Source: CAD feature listing. Evaluate the final solid. Frame: model axes, mm. Give positions to 0.01 mm unless a question says otherwise; leave off trailing zeros. Write each loop counter-clockwise with the first axis right and the second up, starting at its lowest first coordinate (ties: lowest second). Pieces come first, ordered by that corner, then holes. Notation, with made-up numbers: (73.5, 17.5) - (120.5, 17.5) arc R12 ccw to (120.5, 39.5) - close; hole circle Ø4 at (46.25, 23). An arc over 180 degrees is marked (long way). Answer as a JSON object with one key per item and string values. Group by question number.
from build123d import *

# Parameters (mm, degrees)
SKETCH_1_R          = 1.6
EXTRUDE_1_DEPTH     = 2
SKETCH_3_R          = 4.5
SKETCH_3_R_2        = 1.25
CUT_EXTRUDE_1_DEPTH = 3
CUT_EXTRUDE_2_DEPTH = 3
FILLET_1_R          = 1
SKETCH_5_R          = 33.5
CUT_EXTRUDE_3_DEPTH = 3


with BuildPart() as part:
    # ｽｹｯﾁ1 → ﾎﾞｽ - 押し出し1 (new body)
    with BuildSketch(Plane.XY):
        with BuildLine():
            Line((-3, -39.182266397), (-3, -41.291643997))
            Line((-3, -41.291643997), (3, -41.291643997))
            Line((3, -41.291643997), (3, -39.182266397))
            ThreePointArc((3, -39.182266397), (3.498945518, -37.860587373), (4.746835443, -37.198354174))
            ThreePointArc((4.746835443, -37.198354174), (26.516504294, -26.516504294), (37.198354174, -4.746835443))
            ThreePointArc((37.198354174, -4.746835443), (37.860587373, -3.498945518), (39.182266397, -3))
            Line((39.182266397, -3), (41.291643997, -3))
            Line((41.291643997, -3), (41.291643997, 3))
            Line((41.291643997, 3), (39.182266397, 3))
            ThreePointArc((39.182266397, 3), (37.860587373, 3.498945518), (37.198354174, 4.746835443))
            ThreePointArc((37.198354174, 4.746835443), (26.516504294, 26.516504294), (4.746835443, 37.198354174))
            ThreePointArc((4.746835443, 37.198354174), (3.498945518, 37.860587373), (3, 39.182266397))
            Line((3, 39.182266397), (3, 41.291643997))
            Line((3, 41.291643997), (-3, 41.291643997))
            Line((-3, 41.291643997), (-3, 39.182266397))
            ThreePointArc((-3, 39.182266397), (-3.498945518, 37.860587373), (-4.746835443, 37.198354174))
            ThreePointArc((-4.746835443, 37.198354174), (-26.516504294, 26.516504294), (-37.198354174, 4.746835443))
            ThreePointArc((-37.198354174, 4.746835443), (-37.860587373, 3.498945518), (-39.182266397, 3))
            Line((-39.182266397, 3), (-41.291643997, 3))
            Line((-41.291643997, 3), (-41.291643997, -3))
            Line((-41.291643997, -3), (-39.182266397, -3))
            ThreePointArc((-39.182266397, -3), (-37.860587373, -3.498945518), (-37.198354174, -4.746835443))
            ThreePointArc((-37.198354174, -4.746835443), (-26.516504294, -26.516504294), (-4.746835443, -37.198354174))
            ThreePointArc((-4.746835443, -37.198354174), (-3.498945518, -37.860587373), (-3, -39.182266397))
        make_face()
        with Locations((-38.291643997, 0)):
            Circle(SKETCH_1_R, mode=Mode.SUBTRACT)
        with Locations((0, -38.291643997)):
            Circle(SKETCH_1_R, mode=Mode.SUBTRACT)
        with Locations((0, 38.291643997)):
            Circle(SKETCH_1_R, mode=Mode.SUBTRACT)
        with Locations((38.291643997, 0)):
            Circle(SKETCH_1_R, mode=Mode.SUBTRACT)
    extrude(amount=EXTRUDE_1_DEPTH)

    # ｽｹｯﾁ3 → ｶｯﾄ - 押し出し1 (cut, through all)
    with BuildSketch(Plane.XY.offset(2)):
        Circle(SKETCH_3_R)
        with Locations((0, 8.5)):
            Circle(SKETCH_3_R_2)
        with Locations((8.5, 0)):
            Circle(SKETCH_3_R_2)
        with Locations((0, -8.5)):
            Circle(SKETCH_3_R_2)
        with Locations((-8.5, 0)):
            Circle(SKETCH_3_R_2)
    extrude(amount=-CUT_EXTRUDE_1_DEPTH, mode=Mode.SUBTRACT)

    # ｽｹｯﾁ4 → ｶｯﾄ - 押し出し2 (cut, through all)
    with BuildSketch(Plane.XY.offset(2)):
        with BuildLine():
            Line((-3, 33.365401241), (-3, 12.1346611))
            ThreePointArc((-3, 12.1346611), (-8.838834765, 8.838834765), (-12.1346611, 3))
            Line((-12.1346611, 3), (-33.365401241, 3))
            ThreePointArc((-33.365401241, 3), (-23.68807717, 23.68807717), (-3, 33.365401241))
        make_face()
        with BuildLine():
            Line((3, 33.365401241), (3, 12.1346611))
            ThreePointArc((3, 12.1346611), (8.838834765, 8.838834765), (12.1346611, 3))
            Line((12.1346611, 3), (33.365401241, 3))
            ThreePointArc((33.365401241, 3), (23.68807717, 23.68807717), (3, 33.365401241))
        make_face()
        with BuildLine():
            Line((33.365401241, -3), (12.1346611, -3))
            ThreePointArc((12.1346611, -3), (8.838834765, -8.838834765), (3, -12.1346611))
            Line((3, -12.1346611), (3, -33.365401241))
            ThreePointArc((3, -33.365401241), (23.68807717, -23.68807717), (33.365401241, -3))
        make_face()
        with BuildLine():
            Line((-3, -33.365401241), (-3, -12.1346611))
            ThreePointArc((-3, -12.1346611), (-8.838834765, -8.838834765), (-12.1346611, -3))
            Line((-12.1346611, -3), (-33.365401241, -3))
            ThreePointArc((-33.365401241, -3), (-23.68807717, -23.68807717), (-3, -33.365401241))
        make_face()
    extrude(amount=-CUT_EXTRUDE_2_DEPTH, mode=Mode.SUBTRACT)

    # ﾌｨﾚｯﾄ1
    fillet_1_edges = [part.edges().sort_by_distance(p)[0] for p in [
        (-41.291643997, -3, 1),
        (-41.291643997, 3, 1),
        (-3, 41.291643997, 1),
        (3, 41.291643997, 1),
        (41.291643997, 3, 1),
        (41.291643997, -3, 1),
        (3, -41.291643997, 1),
        (-3, -41.291643997, 1),
    ]]
    fillet(fillet_1_edges, radius=FILLET_1_R)

    # ｽｹｯﾁ5 → ｶｯﾄ - 押し出し3 (cut, through all)
    with BuildSketch(Plane.XY.offset(2)):
        Circle(SKETCH_5_R)
    extrude(amount=-CUT_EXTRUDE_3_DEPTH, mode=Mode.SUBTRACT)


solid = part.part
Q1. First-contact query: pin 1 Ø0.6 at (y, z) = (40, 0.5) entering from -X; pin 2 Ø0.9 at (y, z) = (39.5, 0.5) entering from +X; pin 3 Ø0.6 at (x, z) = (39.5, 1.5) entering from -Y. Flat tips, straight axial feed; report the tip coordinate or a pass-through.
Q2. Section A-A on x = 0. Return the cut outline in (y, z), then the cut area to 3 significant figures.
Q3. Section D-D on x = -23.5. Return the cut outline in (y, z).
Q4. Ray query, probe 1 along X at (y, z) = (0.5, 1.1); probe 2 along X at (y, z) = (7, 0.35); probe 3 along X at (y, z) = (9.5, 1.7). Return the intervals inside material, ascending. Write a range as [from, to].
Q5. Section C-C on y = 27. Return the cut outline in (x, z).
Q6. Draft query along Y for faces 1 (the cylindrical face through (37.85, -3.51, 0.99)), 2 (the flat face through (0, 41.292, 1)), 3 (the cylindrical face through (-0.208, 39.878, 0.986)), 4 (the cylindrical face through (0.74, -39.71, 0.99)). Return one class per face: released by +Y, released by -Y, zero draft, split by the parting line, or undercut.
Taken from the geometry:
{
 "1": {"pin 1": "stops at x = -3", "pin 2": "stops at x = 3", "pin 3": "stops at y = -3"},
 "2": {"outline": "(-41.29, 0) - (-39.89, 0) - (-39.89, 2) - (-41.29, 2) - close; (-36.69, 0) - (-33.5, 0) - (-33.5, 2) - (-36.69, 2) - close; (33.5, 0) - (36.69, 0) - (36.69, 2) - (33.5, 2) - close; (39.89, 0) - (41.29, 0) - (41.29, 2) - (39.89, 2) - close", "area": "18.4 mm²"},
 "3": {"outline": "(-29.22, 0) - (-23.87, 0) - (-23.87, 2) - (-29.22, 2) - close; (23.87, 0) - (29.22, 0) - (29.22, 2) - (23.87, 2) - close"},
 "4": {"probe 1": "x = [-41.29, -39.81], [-36.77, -33.5], [33.5, 36.77], [39.81, 41.29]", "probe 2": "x = [-36.84, -32.76], [32.76, 36.84]", "probe 3": "x = [-36.28, -32.12], [32.12, 36.28]"},
 "5": {"outline": "(-26.02, 0) - (-19.83, 0) - (-19.83, 2) - (-26.02, 2) - close; (19.83, 0) - (26.02, 0) - (26.02, 2) - (19.83, 2) - close"},
 "6": {"face 1": "released by -Y", "face 2": "released by +Y", "face 3": "undercut", "face 4": "undercut"}
}
